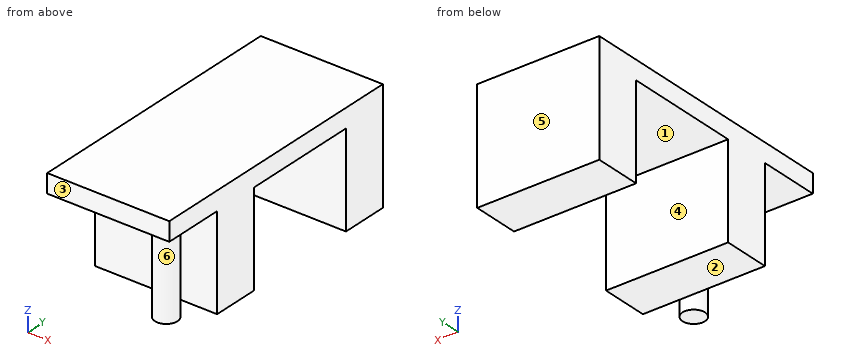
```python
from build123d import *

# Parameters (mm, degrees)
SKETCH082_W  = 26
SKETCH082_H  = 58
PAD036_DEPTH = 4
SKETCH083_W  = 26
SKETCH083_H  = 10
PAD037_DEPTH = 20
SKETCH084_R  = 2.4
PAD038_DEPTH = 17


with BuildPart() as part:
    # Sketch082 → Pad036 (new body)
    with BuildSketch(Plane(origin=(125, -105, 16), x_dir=(1, 0, 0), z_dir=(0, 0, -1))):
        with Locations((5, 1)):
            Rectangle(SKETCH082_W, SKETCH082_H)
    extrude(amount=PAD036_DEPTH)

    # Sketch083 → Pad037 (new body)
    with BuildSketch(Plane(origin=(125, -105, 12), x_dir=(1, 0, 0), z_dir=(0, 0, -1))):
        with Locations((5, 12)):
            Rectangle(SKETCH083_W, SKETCH083_H)
        with Locations((5, -23)):
            Rectangle(SKETCH083_W, SKETCH083_H)
    extrude(amount=PAD037_DEPTH)

    # Sketch084 → Pad038 (new body)
    with BuildSketch(Plane(origin=(125, -105, 12), x_dir=(1, 0, 0), z_dir=(0, 0, -1))):
        with Locations((15, 27)):
            Circle(SKETCH084_R)
    extrude(amount=PAD038_DEPTH)


solid = part.part
```
Build history of the part. All positions in model axes, mm. Face numbers are marked on the shaded views. A direction names the side the tool comes from. Give positions to 0.01 mm unless a question says otherwise; leave off trailing zeros. Loops run counter-clockwise (first coordinate to the right, second up) from the corner with the lowest first, then second, coordinate; pieces in that order, holes last.
Item 1: Flat gauge pins, fed straight in: pin 1 (7.5 mm diameter, centred on x = 129.5, y = -98.5, fed in from -Z); pin 2 (6 mm diameter, centred on x = 126.5, z = 7, fed in from -Y); pin 3 (2.5 mm diameter, centred on x = 141, y = -132.5, fed in from -Z). Where does each tip first touch, or does it go through?
Answers follow:
pin 1: stops at z = 12
pin 2: stops at y = -122
pin 3: stops at z = -5
Item 2: Pull direction Y, two halves, no side cores. Call the marked faces 1, 2 and 3: released by +Y, released by -Y, zero draft, split by the parting line, or undercut.
Answers follow:
face 1: undercut
face 2: zero draft
face 3: released by -Y
Item 3: Slice it at D-D, the plane x = 121. List the corners of the cut face in (y, z), and give its area (3 significant figures).
Answers follow:
outline: (-135, 12) - (-122, 12) - (-122, -8) - (-112, -8) - (-112, 12) - (-87, 12) - (-87, -8) - (-77, -8) - (-77, 16) - (-135, 16) - close
area: 632 mm2
Item 4: Which spindle directions (+Z, -Z, +X, -X, +Y, -Y) get a long thin tool onto all of the face, cutting with end or side? Do the marked faces 4, 5 and 6. Say none if no direction does.
Answers follow:
face 4: -Z, +X, -X
face 5: +Z, -Z, +X, -X, +Y
face 6: -Z
Item 5: Drill centre lines: line 1 (Y direction, x = 128.25, z = 11); line 2 (Z direction, x = 127.75, y = -90); line 3 (X direction, y = -130.5, z = 3). Where is each one in solid material? Low to high.
Answers follow:
line 1: y = -122 to -112, -87 to -77
line 2: z = 12 to 16
line 3: x = 138.13 to 141.87
Item 6: Slice it at A-A, the plane z = 8.75. List the corners of the cut face in (x, y), and give its area (3 significant figures).
Answers follow:
outline: (117, -122) - (143, -122) - (143, -112) - (117, -112) - close; (117, -87) - (143, -87) - (143, -77) - (117, -77) - close; circle Ø4.8 at (140, -132)
area: 538 mm2
Item 7: Slice it at B-B, the plane x = 140. List the corners of the cut face in (y, z), and give its area (3 significant figures).
Answers follow:
outline: (-135, 12) - (-134.4, 12) - (-134.4, -5) - (-129.6, -5) - (-129.6, 12) - (-122, 12) - (-122, -8) - (-112, -8) - (-112, 12) - (-87, 12) - (-87, -8) - (-77, -8) - (-77, 16) - (-135, 16) - close
area: 714 mm2
Item 8: Slice it at C-C, the plane y = -132. List the corners of the cut face in (x, z).
Answers follow:
outline: (117, 12) - (137.6, 12) - (137.6, -5) - (142.4, -5) - (142.4, 12) - (143, 12) - (143, 16) - (117, 16) - close
